from build123d import *

# Parameters (mm, degrees)
BOSS_EXTRUDE1_DEPTH      = 279.4
BOSS_EXTRUDE1_DEPTH_BACK = 279.4
SKETCH5_R                = 3.175
CUT_EXTRUDE1_DEPTH       = 281.839473721
SKETCH6_R                = 19.05
CUT_EXTRUDE2_DEPTH       = 455.280260412


with BuildPart() as part:
    # Sketch4 → Boss-Extrude1 (new, two sides: drawn at the far end of the back side and taken through both)
    with BuildSketch(Plane(origin=(0, 0, 0), x_dir=(0, 0, -1), z_dir=(1, 0, 0)).offset(-BOSS_EXTRUDE1_DEPTH_BACK)):
        with BuildLine():
            Line((12.7, -11.43), (12.7, 11.43))
            ThreePointArc((12.7, 11.43), (12.328025612, 12.328025612), (11.43, 12.7))
            Line((11.43, 12.7), (-11.43, 12.7))
            ThreePointArc((-11.43, 12.7), (-12.328025612, 12.328025612), (-12.7, 11.43))
            Line((-12.7, 11.43), (-12.7, -11.43))
            ThreePointArc((-12.7, -11.43), (-12.328025612, -12.328025612), (-11.43, -12.7))
            Line((-11.43, -12.7), (11.43, -12.7))
            ThreePointArc((11.43, -12.7), (12.328025612, -12.328025612), (12.7, -11.43))
        make_face()
        with BuildLine():
            Line((11.049, 9.9441), (11.049, -9.9441))
            ThreePointArc((11.049, -9.9441), (10.725382283, -10.725382283), (9.9441, -11.049))
            Line((9.9441, -11.049), (-9.9441, -11.049))
            ThreePointArc((-9.9441, -11.049), (-10.725382283, -10.725382283), (-11.049, -9.9441))
            Line((-11.049, -9.9441), (-11.049, 9.9441))
            ThreePointArc((-11.049, 9.9441), (-10.725382283, 10.725382283), (-9.9441, 11.049))
            Line((-9.9441, 11.049), (9.9441, 11.049))
            ThreePointArc((9.9441, 11.049), (10.725382283, 10.725382283), (11.049, 9.9441))
        make_face(mode=Mode.SUBTRACT)
    extrude(amount=BOSS_EXTRUDE1_DEPTH + BOSS_EXTRUDE1_DEPTH_BACK)

    # Sketch5 → Cut-Extrude1 (cut, through all)
    with BuildSketch(Plane.XY.offset(12.7)):
        with Locations((-266.7, 0)):
            Circle(SKETCH5_R)
    extrude(amount=-CUT_EXTRUDE1_DEPTH, mode=Mode.SUBTRACT)

    # Sketch6 → Cut-Extrude2 (cut, through all)
    with BuildSketch(Plane(origin=(146.05, 146.05, 0), x_dir=(0, 0, 1), z_dir=(0.7071067811865464, 0.7071067811865488, 0))):
        with Locations((0, 203.243890785)):
            Circle(SKETCH6_R)
    extrude(amount=-CUT_EXTRUDE2_DEPTH, mode=Mode.SUBTRACT)


solid = part.part
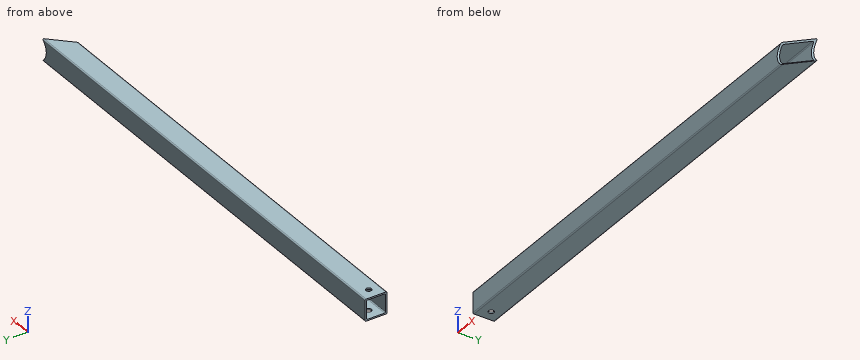
Geometry check sheet. Reference: the model listing, model coordinates, mm. Round coordinates to 2 decimals unless told otherwise and drop trailing zeros. Write each loop counter-clockwise with the first axis right and the second up, starting at its lowest first coordinate (ties: lowest second). Pieces come first, ordered by that corner, then holes. Notation, with made-up numbers: (-16.5, 62.25) -> (5.5, 62.25) arc R31 cw to (5.5, 98.25) -> close; hole circle Ø2 at (88, 58.5). An arc over 180 degrees is marked (long way). One line per item, written item: value. Start each with the question number.
(1) Scan lines: line 1 (Z direction, x = -2, y = 2); line 2 (Y direction, x = -266.7, z = -11.85) (3 decimals); line 3 (Y direction, x = -266.7, z = -11.5) (3 decimals). Record each from-to range of solid material in increasing order. Write a range as [from, to].
(2) Go/stop test with a flat-tipped pin: pin 1 Ø8.5 at (x, y) = (-266.7, 0) entering from -Z. Record where the tip stops, or that it passes through.
(3) Cross-section at B-B, the plane x = -113.5. Record the cut outline in (y, z), and give its area (3 significant figures).
(4) Cross-section at A-A, the plane z = -0.5. Record the cut outline in (x, y).
Answer:
1. line 1: [-12.7, -11.05], [11.05, 12.7]
1. line 2: [-12.629, -3.175], [3.175, 12.629]
1. line 3: [-12.698, -3.175], [3.175, 12.698]
2. pin 1: z = -12.7
3. outline: (-12.7, -11.43) arc R1.27 ccw to (-11.43, -12.7) -> (11.43, -12.7) arc R1.27 ccw to (12.7, -11.43) -> (12.7, 11.43) arc R1.27 ccw to (11.43, 12.7) -> (-11.43, 12.7) arc R1.27 ccw to (-12.7, 11.43) -> close; hole (-11.05, -9.94) arc R1.1 ccw to (-9.94, -11.05) -> (9.94, -11.05) arc R1.1 ccw to (11.05, -9.94) -> (11.05, 9.94) arc R1.1 ccw to (9.94, 11.05) -> (-9.94, 11.05) arc R1.1 ccw to (-11.05, 9.94) -> close
3. area: 157 mm²
4. outline: (-279.4, -12.7) -> (247.8, -12.7) -> (249.45, -11.05) -> (-279.4, -11.05) -> close; (-279.4, 11.05) -> (271.55, 11.05) -> (273.2, 12.7) -> (-279.4, 12.7) -> close
